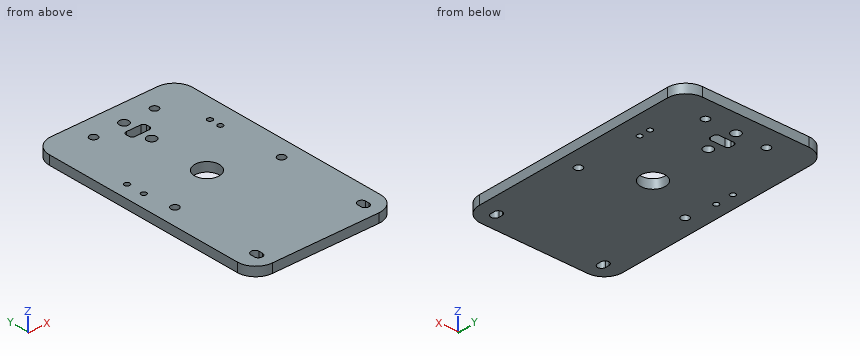
from build123d import *

# Parameters (mm, degrees)
MODEL_R           = 3.1
MODEL_R_2         = 2.6
MODEL_W           = 13.5
MODEL_H           = 6.2
BASE_DEPTH        = 6
SKETCH_1_R        = 8.05
BEARINGHOLE_DEPTH = 10
SKETCH1_R         = 1.75
SENSORMOUNT_DEPTH = 10
SKETCH3_R         = 1.75
CABLEMOUNT_DEPTH  = 10
FILLETCABLESLOT_R = 2


with BuildPart() as part:
    # Model → Base (new body)
    with BuildSketch(Plane.XY):
        with BuildLine():
            Line((-35, 160), (35, 160))
            ThreePointArc((35, 160), (43.485281374, 156.485281374), (47, 148))
            Line((47, 148), (47, 12))
            ThreePointArc((47, 12), (43.485281374, 3.514718626), (35, 0))
            Line((35, 0), (-35, 0))
            ThreePointArc((-35, 0), (-43.485281374, 3.514718626), (-47, 12))
            Line((-47, 12), (-47, 148))
            ThreePointArc((-47, 148), (-43.485281374, 156.485281374), (-35, 160))
        make_face()
        with Locations((0, 145.8)):
            Circle(MODEL_R, mode=Mode.SUBTRACT)
        with Locations((-20, 145.8)):
            Circle(MODEL_R_2, mode=Mode.SUBTRACT)
        with Locations((20, 145.8)):
            Circle(MODEL_R_2, mode=Mode.SUBTRACT)
        with Locations((-35, 70.45)):
            Circle(MODEL_R_2, mode=Mode.SUBTRACT)
        with Locations((0, 125.8)):
            Circle(MODEL_R, mode=Mode.SUBTRACT)
        with Locations((35, 70.45)):
            Circle(MODEL_R_2, mode=Mode.SUBTRACT)
        with BuildLine():
            Line((-32.4, 12.5), (-32.4, 10))
            ThreePointArc((-32.4, 10), (-35, 7.4), (-37.6, 10))
            Line((-37.6, 10), (-37.6, 12.5))
            ThreePointArc((-37.6, 12.5), (-35, 15.1), (-32.4, 12.5))
        make_face(mode=Mode.SUBTRACT)
        with BuildLine():
            Line((32.4, 12.5), (32.4, 10))
            ThreePointArc((32.4, 10), (35, 7.4), (37.6, 10))
            Line((37.6, 10), (37.6, 12.5))
            ThreePointArc((37.6, 12.5), (35, 15.1), (32.4, 12.5))
        make_face(mode=Mode.SUBTRACT)
        with Locations((0, 135.8)):
            Rectangle(MODEL_W, MODEL_H, mode=Mode.SUBTRACT)
    extrude(amount=BASE_DEPTH)

    # Эскиз1 → BearingHole (cut)
    with BuildSketch(Plane(origin=(0, 0, 0), x_dir=(-1, 0, 0), z_dir=(0, 0, -1))):
        with Locations((0, 85.8)):
            Circle(SKETCH_1_R)
    extrude(amount=-BEARINGHOLE_DEPTH, mode=Mode.SUBTRACT)

    # Sketch1 → SensorMount (cut)
    with BuildSketch(Plane.XY.offset(6)):
        with Locations((33, 120)):
            Circle(SKETCH1_R)
        with Locations((33, 112.5)):
            Circle(SKETCH1_R)
    extrude(amount=-SENSORMOUNT_DEPTH, mode=Mode.SUBTRACT)

    # Sketch3 → CableMount (cut)
    with BuildSketch(Plane(origin=(0, 0, 0), x_dir=(-1, 0, 0), z_dir=(0, 0, -1))):
        with Locations((37.6, 90.08855339)):
            Circle(SKETCH3_R)
        with Locations((37.6, 102.08855339)):
            Circle(SKETCH3_R)
    extrude(amount=-CABLEMOUNT_DEPTH, mode=Mode.SUBTRACT)

    # FilletCableSlot
    filletcableslot_edges = [part.edges().sort_by_distance(p)[0] for p in [
        (6.75, 132.7, 3),
        (6.75, 138.9, 3),
        (-6.75, 138.9, 3),
        (-6.75, 132.7, 3),
    ]]
    fillet(filletcableslot_edges, radius=FILLETCABLESLOT_R)


solid = part.part
Read the model definition and answer for the solid it produces. Units are mm, in the model's axes. Give positions to 0.01 mm unless a question says otherwise; leave off trailing zeros. Write each loop counter-clockwise with the first axis right and the second up, starting at its lowest first coordinate (ties: lowest second). Pieces come first, ordered by that corner, then holes. Notation, with made-up numbers: (-33, 50.25) - (15, 50.25) arc R27 ccw to (15, 74.25) - close; hole circle Ø11 at (63, 69). An arc over 180 degrees is marked (long way). Use CSV: the item, a comma, the result in double quotes. Start each with the question number.
(1) Find section D-D (z = 3.3). Count the separate pieces of the cut face and the enclosed holes in it, plus the area to 3 significant figures.
(2) Consider line 1 along X through (y, z) = (145.8, 1.55); line 2 along Y through (x, z) = (35, 2.25); line 3 along Y through (x, z) = (-20, 4.3). Determine where each line is inside the solid, lowest interval first.
(3) Find section B-B (y = 125.8). Give the vertices of the cut face in (x, z), plus the area to 3 significant figures.
(4) Find section C-C (y = 85.8). Give the vertices of the cut face in (x, z).
(5) Find section A-A (y = 145.8). Give the vertices of the cut face in (x, z), plus the area to 3 significant figures.
Findings below:
1,separate pieces,"1"
1,enclosed holes,"14"
1,area,"14,400 mm2"
2,line 1,"-47 to -22.6, -17.4 to -3.1, 3.1 to 17.4, 22.6 to 47"
2,line 2,"0 to 7.4, 15.1 to 67.85, 73.05 to 160"
2,line 3,"0 to 143.2, 148.4 to 160"
3,outline,"(-47, 0) - (-3.1, 0) - (-3.1, 6) - (-47, 6) - close; (3.1, 0) - (47, 0) - (47, 6) - (3.1, 6) - close"
3,area,"527 mm2"
4,outline,"(-47, 0) - (-8.05, 0) - (-8.05, 6) - (-47, 6) - close; (8.05, 0) - (47, 0) - (47, 6) - (8.05, 6) - close"
5,outline,"(-47, 0) - (-22.6, 0) - (-22.6, 6) - (-47, 6) - close; (-17.4, 0) - (-3.1, 0) - (-3.1, 6) - (-17.4, 6) - close; (3.1, 0) - (17.4, 0) - (17.4, 6) - (3.1, 6) - close; (22.6, 0) - (47, 0) - (47, 6) - (22.6, 6) - close"
5,area,"464 mm2"
